Design review of the part built by this model. Coordinates are the model's own, in mm. Face numbers are marked on the shaded views. A direction names the side the tool comes from. Give positions to 0.01 mm unless a question says otherwise; leave off trailing zeros. Write each loop counter-clockwise with the first axis right and the second up, starting at its lowest first coordinate (ties: lowest second). Pieces come first, ordered by that corner, then holes. Notation, with made-up numbers: M 65,17 L 82,17 A24 ccw 82,47 Z; hole C -22.75,-10.75 d11. An arc over 180 degrees is marked long. One line per item, written item: value. Start each with the question number.
```python
from build123d import *

# Parameters (mm, degrees)
SKETCH1_R                       = 57.15
BOSS_EXTRUDE1_DEPTH             = 63.5
SKETCH2_R                       = 41.275
CUT_EXTRUDE1_DEPTH              = 53.34
F_1_4_0_25_DIAMETER_HOLE4_D     = 6.35
F_1_4_0_25_DIAMETER_HOLE4_DEPTH = 25.4
F_1_4_0_25_DIAMETER_HOLE4_TIP   = 1.907732465
SKETCH7_R                       = 3.81
CUT_EXTRUDE2_DEPTH              = 103.783729257
F_4_0MM_DOWEL_HOLE1_D           = 4
SKETCH9_W                       = 7
SKETCH9_H                       = 7
CUT_EXTRUDE3_DEPTH              = 3.5
SKETCH12_W                      = 12.7
SKETCH12_H                      = 19.05
CUT_EXTRUDE4_DEPTH              = 4.7625


with BuildPart() as part:
    # Sketch1 → Boss-Extrude1 (new body)
    with BuildSketch(Plane(origin=(0, 0, 0), x_dir=(1, 0, 0), z_dir=(0, 1, 0))):
        with Locations(Location((0, 0, 0), (0, 0, 270))):
            Circle(SKETCH1_R)
    extrude(amount=BOSS_EXTRUDE1_DEPTH)

    # Sketch2 → Cut-Extrude1 (cut)
    with BuildSketch(Plane(origin=(0, 63.5, 0), x_dir=(1, 0, 0), z_dir=(0, 1, 0))):
        with Locations(Location((0, 0, 0), (0, 0, 270))):
            Circle(SKETCH2_R)
    extrude(amount=-CUT_EXTRUDE1_DEPTH, mode=Mode.SUBTRACT)

    # 1/4 (0.25) Diameter Hole4
    with Locations(Plane(origin=(0, 63.5, 0), x_dir=(1, 0, 0), z_dir=(0, 1, 0))):
        with Locations((-41.244459855, 23.8125), (0, -47.625), (41.244459855, 23.8125)):
            Hole(F_1_4_0_25_DIAMETER_HOLE4_D / 2, depth=F_1_4_0_25_DIAMETER_HOLE4_DEPTH)
            with Locations((0, 0, -(F_1_4_0_25_DIAMETER_HOLE4_DEPTH + F_1_4_0_25_DIAMETER_HOLE4_TIP / 2))):  # 118° drill point
                Cone(0, F_1_4_0_25_DIAMETER_HOLE4_D / 2, F_1_4_0_25_DIAMETER_HOLE4_TIP, mode=Mode.SUBTRACT)

    # Sketch7 → Cut-Extrude2 (cut, through all)
    with BuildSketch(Plane.XY):
        with Locations((0, 15.24)):
            Circle(SKETCH7_R)
    extrude(amount=-CUT_EXTRUDE2_DEPTH, mode=Mode.SUBTRACT)

    # Ø4.0mm Dowel Hole1 (through all)
    with Locations(Plane(origin=(-5, 0, 15.938504039), x_dir=(0, 0, -1), z_dir=(0, -1, 0))):
        with Locations((0, 0), (0, 10), (49.5, 10), (49.5, 0)):
            Hole(F_4_0MM_DOWEL_HOLE1_D / 2)

    # Sketch9 → Cut-Extrude3 (cut)
    with BuildSketch(Plane.XZ):
        with Locations((-5, 15.938504039)):
            Rectangle(SKETCH9_W, SKETCH9_H)
        with Locations((5, 15.938504039)):
            Rectangle(SKETCH9_W, SKETCH9_H)
        with Locations((5, -33.561495961)):
            Rectangle(SKETCH9_W, SKETCH9_H)
        with Locations((-5, -33.561495961)):
            Rectangle(SKETCH9_W, SKETCH9_H)
    extrude(amount=-CUT_EXTRUDE3_DEPTH, mode=Mode.SUBTRACT)

    # Sketch12 → Cut-Extrude4 (cut)
    with BuildSketch(Plane(origin=(0, 50.8, 0), x_dir=(1, 0, 0), z_dir=(0, 1, 0))):
        Polygon((-54.992429237, 24.417545405), (-38.494645295, 14.892545405), (-35.319645295, 20.391806719), (-51.817429237, 29.916806719), align=None)
        Polygon((-51.817429237, 29.916806719), (-35.319645295, 20.391806719), (-32.144645295, 25.891068033), (-48.642429237, 35.416068033), align=None)
        Polygon((32.144645295, 25.891068033), (35.319645295, 20.391806719), (51.817429237, 29.916806719), (48.642429237, 35.416068033), align=None)
        Polygon((51.817429237, 29.916806719), (35.319645295, 20.391806719), (38.494645295, 14.892545405), (54.992429237, 24.417545405), align=None)
        with Locations((0, -50.308613437)):
            Rectangle(SKETCH12_W, SKETCH12_H)
    extrude(amount=CUT_EXTRUDE4_DEPTH, mode=Mode.SUBTRACT)


solid = part.part
```
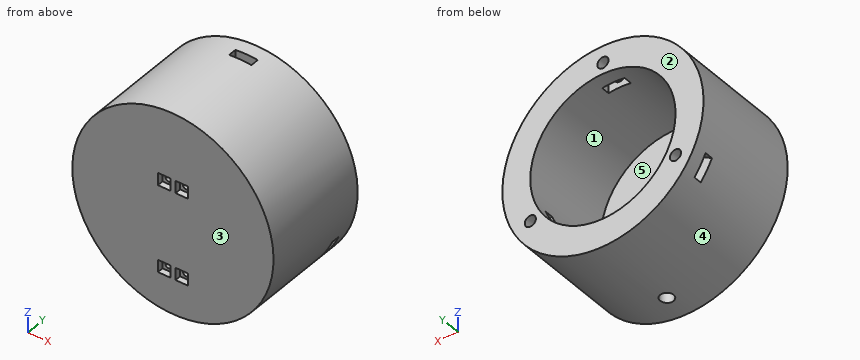
Q1. Wall thickness on line 1 (Z direction, x = 0, y = 39) (3 decimals); line 2 (X direction, y = 59.5, z = 46); line 3 (Z direction, x = -34, y = 23.5): over which ranges is each line inside the solid? List them lowest first. Write a range as from..to.
Q2. Take a section at B-B, the plane z = 0. Give the boundary of the cut face in (x, y) (3 decimals), then the cut area to 3 significant figures.
Q3. Take a section at A-A, the plane y = 53. Give the boundary of the cut face in (x, z) (3 decimals).
Q4. Take a section at D-D, the plane y = 29. Give the boundary of the cut face in (x, z) (3 decimals), then the cut area to 3 significant figures.
Q5. The part is to be moulded in two halves that separate along Z. For the marked faces 3, 4 and 5, say which applies: pulls with the +Z half, pulls with the -Z half, needs draft (parallel to the pull), parting line crosses it, or undercut.
Q6. Machinability: for the marked faces 1 and 2, which of the approach directions +Z, -Z, +X, -X, +Y, -Y give a long, thin tool a straight path to every point of the face, cutting with its end or side? Answer none if there is none.
Q7. For P1, Ø6, axis at y = 47, z = 18, coming from the +X side; P2, Ø12, axis at y = 48, z = -8, coming from the +X side (3 decimals); P3, Ø3, axis at x = -6.5, y = 1.5, coming from the +Z side; P4, Ø2.5, axis at x = 5, z = -33.56, coming from the +Y side, all flat-tipped, find the tip position at first contact; note any pin that passes through.
Q8. Take a section at C-C, the plane x = -18. Give the boundary of the cut face in (y, z), then the cut area to 3 significant figures.
Results list:
1. line 1: z = -57.15..-41.275, 41.275..44.45, 50.8..57.15
1. line 2: x = -33.91..-2.73, 2.73..33.91
1. line 3: z = -45.94..-23.4, 23.4..45.94
2. outline: M -57.15,0 L 57.15,0 L 57.15,63.5 L 41.275,63.5 L 41.275,10.16 L -41.275,10.16 L -41.275,63.5 L -57.15,63.5 Z
2. area: 2,850 mm^2
3. outline: M -52.362,-22.899 L -38.495,-14.893 A41.275 cw -6.35,40.784 L -6.35,56.796 A57.15 ccw Z; M -46.012,-33.897 A57.15 ccw 46.012,-33.897 L 32.145,-25.891 A41.275 cw -32.145,-25.891 Z; M 6.35,40.784 A41.275 cw 38.495,-14.893 L 52.362,-22.899 A57.15 ccw 6.35,56.796 Z
4. outline: C 0,0 d114.3; hole C 0,0 d82.55
4. area: 4,910 mm^2
5. face 3: needs draft
5. face 4: parting line crosses it
5. face 5: undercut
6. face 1: +Y
6. face 2: +Z, -Z, +X, -X, +Y
7. P1: stops at x = 55.15
7. P2: stops at x = 57.115
7. P3: stops at z = 56.93
7. P4: passes through
8. outline: M 0,-54.24 L 63.5,-54.24 L 63.5,-37.14 L 10.16,-37.14 L 10.16,37.14 L 63.5,37.14 L 63.5,54.24 L 0,54.24 Z
8. area: 2,930 mm^2
